Input: part model. Units: mm. Frame: model coordinates. Face numbers are marked on the shaded views. A direction names the side the tool comes from. Give positions to 0.01 mm unless a question says otherwise; leave off trailing zeros. Loops run counter-clockwise (first coordinate to the right, second up) from the corner with the lowest first, then second, coordinate; pieces in that order, holes last. Notation, with made-up numbers: M -33,85 L 17,85 A31 cw 17,120 Z; hole C 38,-16.75 d1. An arc over 180 degrees is marked long. One line per item, written item: value. Start each with the question number.
(1) Pin query (flat end, axial travel): P1, Ø15.5, axis at x = -89, z = -76.5, coming from the +Y side; P2, Ø3, axis at x = 54.5, z = 112.5, coming from the +Y side; P3, Ø12.5, axis at x = 60, y = 17, coming from the +Z side. Return the tip coordinate at first contact, or that it passes through.
(2) Pull-direction query (Y, two-part tool) for the marked faces 4, 5 and 6; classes: released by +Y, released by -Y, zero draft, split by the parting line, or undercut.
(3) Ray query, line 1 along Y through (x, z) = (0, 86); line 2 along Y through (x, z) = (3, 50); line 3 along Z through (x, y) = (-33, -5.5). Return the intervals inside material, ascending. Write a range as from..to.
(4) Section A-A on y = -131.5. Output: boundary loops of the cut face in (x, z), plus the area to 3 significant figures.
(5) Section B-B on z = -70.5. Output: boundary loops of the cut face in (x, y).
(6) Access query for the marked faces 1, 2 and 3. Directions: +Z, -Z, +X, -X, +Y, -Y. A direction counts if a zero-diameter tool reaches every point of the face in a straight line with its end or side. Return the directions, or none.
(7) Section D-D on y = 121.5. Output: boundary loops of the cut face in (x, z).
(8) Section C-C on x = 115.5. Output: boundary loops of the cut face in (y, z), plus the area to 3 significant figures.
```python
from build123d import *

# Parameters (mm, degrees)
F0_R           = 152.4
F1_DEPTH       = 203.2
F2_R           = 88.9
F3_DEPTH       = 254
F4_W           = 118.0947571993
F4_H           = 79.6899646521
F5_DEPTH       = 152.4
F5_TAPER       = 3
F6_W           = 94.8493182659
F6_H           = 110.4671433568
F7_DEPTH       = 325.12
F8_R           = 142.764871417
F9_DEPTH       = 152.4
F10_W          = 79.6899646521
F10_H          = 52.806597203
F11_DEPTH      = 101.6
F11_DEPTH_BACK = 101.6
F13_DEPTH      = 127
F13_DEPTH_BACK = 127
F15_DEPTH      = 101.6
F15_DEPTH_BACK = 101.6
F17_DEPTH      = 322.505


with BuildPart() as f1:
    # F0 (on Top) → F1 (new body)
    with BuildSketch(Plane.XY):
        Circle(F0_R)
    extrude(amount=F1_DEPTH)

    # F2 (on face) → F3 (join)
    with BuildSketch(Plane(origin=(0, 0, 0), x_dir=(1, 0, 0), z_dir=(0, 0, -1))):
        Circle(F2_R)
    extrude(amount=F3_DEPTH)

    # F4 (on Front) → F5 (cut)
    with BuildSketch(Plane.XZ):
        with Locations((0.4800595343, -158.3820804954)):
            Rectangle(F4_W, F4_H)
    extrude(amount=F5_DEPTH, taper=F5_TAPER, mode=Mode.SUBTRACT)

    # F6 (on face) → F7 (cut)
    with BuildSketch(Plane.XY.offset(203.2)):
        Rectangle(F6_W, F6_H)
    extrude(amount=-F7_DEPTH, mode=Mode.SUBTRACT)

    # F8 (on face) → F9 (cut)
    with BuildSketch(Plane.XY.offset(203.2)):
        Circle(F8_R)
    extrude(amount=-F9_DEPTH, mode=Mode.SUBTRACT)

    # F10 (on Right) → F11 (cut, two sides)
    with BuildSketch(Plane.YZ) as f11_sk:
        with Locations((6.1672367156, -58.5296023637)):
            Rectangle(F10_W, F10_H)
    extrude(amount=F11_DEPTH, mode=Mode.SUBTRACT)
    extrude(f11_sk.sketch, amount=-F11_DEPTH_BACK, mode=Mode.SUBTRACT)

    # F12 (on Right) → F13 (join, two sides)
    with BuildSketch(Plane.YZ) as f13_sk:
        Polygon((45.9540584598, -31.9147333503), (-33.2359305319, -31.9147333503), (-45.800998807, -59.6464499831), (57.6868057251, -59.6464499831), align=None)
    extrude(amount=F13_DEPTH)
    extrude(f13_sk.sketch, amount=-F13_DEPTH_BACK)

    # F14 (on Right) → F15 (join, two sides)
    with BuildSketch(Plane.YZ) as f15_sk:
        Polygon((-33.7745137513, -59.7862656422), (-40.2827188373, -59.6054829657), (-33.7745137513, -85.3911563754), align=None)
        Polygon((53.6378957331, -59.6221797168), (45.722966075, -59.6221797168), (45.800998807, -85.1639956236), align=None)
    extrude(amount=F15_DEPTH)
    extrude(f15_sk.sketch, amount=-F15_DEPTH_BACK)

    # F16 (on Front) → F17 (join)
    with BuildSketch(Plane.XZ):
        Polygon((58.3297610283, -193.6283260584), (-52.9678873718, -193.6283260584), (-52.9678873718, -254.0221810341), (58.3297610283, -252.9366910458), align=None)
    extrude(amount=F17_DEPTH)


solid = f1.part
```
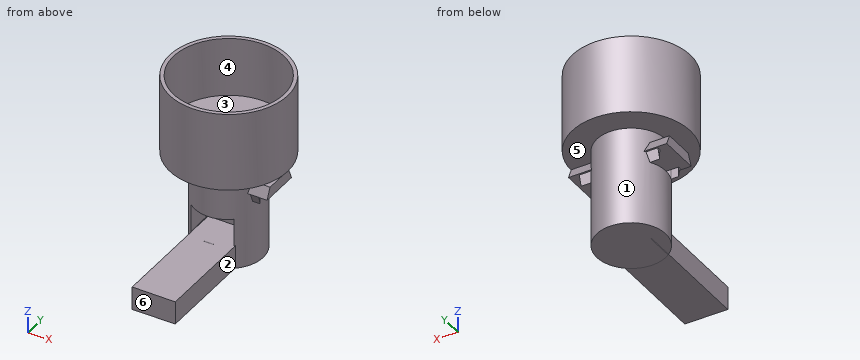
Output values:
1. P1: stops at y = 50.84
1. P2: stops at y = 142.89
1. P3: stops at z = 50.8
2. face 4: undercut
2. face 5: zero draft
2. face 6: released by -Y
3. line 1: y = -152.4..-142.76, 142.76..152.4
3. line 2: y = -152.37..-55.23, 55.23..152.37
3. line 3: z = -254..-193.63, -59.65..-31.91
4. outline: M -77.03,0 L 77.03,0 L 77.03,203.2 L 55.58,203.2 L 55.58,50.8 L -55.58,50.8 L -55.58,203.2 L -77.03,203.2 Z; M -52.97,-254.02 L 58.33,-252.94 L 58.33,-193.63 L -52.97,-193.63 Z
4. area: 21,000 mm²
5. outline: M -101.6,-37.53 L -80.59,-37.53 A88.9 ccw 80.59,-37.53 L 101.6,-37.53 L 101.6,-33.77 L 82.23,-33.77 A88.9 ccw 82.27,-33.68 L 47.42,-33.68 L 47.42,-33.77 L -47.42,-33.77 L -47.42,-33.68 L -82.27,-33.68 A88.9 ccw -82.23,-33.77 L -101.6,-33.77 Z; M -101.6,45.76 L 101.6,45.76 L 101.6,50.3 L 73.3,50.3 A88.9 ccw -73.3,50.3 L -101.6,50.3 Z; hole M -47.42,-55.23 L 47.42,-55.23 L 47.42,-37.53 L -47.42,-37.53 Z; hole M -47.42,50.3 L 47.42,50.3 L 47.42,55.23 L -47.42,55.23 Z
6. face 1: none
6. face 2: -Z, +X, -Y
6. face 3: +Z
7. outline: M -92,0 L 92,0 L 92,203.2 L 74.96,203.2 L 74.96,50.8 L -74.96,50.8 L -74.96,203.2 L -92,203.2 Z
8. outline: M -99.43,0 L 99.43,0 L 99.43,203.2 L 83.91,203.2 L 83.91,50.8 L -83.91,50.8 L -83.91,203.2 L -99.43,203.2 Z; M -45.8,-59.65 L 57.69,-59.65 L 45.95,-31.91 L -33.24,-31.91 Z
8. area: 17,400 mm²
